The model under review builds one solid part; all positions refer to its coordinate system, in mm. A direction names the side the tool comes from. Round coordinates to 2 decimals unless told otherwise and drop trailing zeros. Order: outer loops, then holes, each group sorted by start corner. A loop starts at its lowest first (then second) coordinate and runs counter-clockwise, first axis right, second up.
Autodesk Inventor part; units mm, degrees
ref_plane "YZ Plane" through (0, 0, 0) normal (1, 0, 0) x (0, 1, 0)
ref_plane "XZ Plane" through (0, 0, 0) normal (0, 1, 0) x (-1, 0, 0)
ref_plane "XY Plane" through (0, 0, 0) normal (0, 0, 1) x (1, 0, 0)
sketch "Эскиз1" plane through (0, 0, 0) normal (0, 1, 0) x (-1, 0, 0)
  circle A0 centre (0, 8.5) radius 1.3
  circle A1 centre (0, -8.5) radius 1.3
  line L0 (0, 5.7) -> (3, 5.7)
  line L1 (3, 5.7) -> (3, 11.7)
  line L2 (3, 11.7) -> (-10, 11.7)
  line L3 (-10, 11.7) -> (-10, 0)
  line L4 (5.8356, 0) -> (-16.6075, 0) construction
  line L5 (0, 5.7) -> (0, 0)
  circle A2 centre (0, -8.5) radius 1.3
  line L6 (0, -5.7) -> (3, -5.7)
  line L7 (3, -5.7) -> (3, -11.7)
  line L8 (3, -11.7) -> (-10, -11.7)
  line L9 (-10, -11.7) -> (-10, 0)
  line L10 (0, -5.7) -> (0, 0)
  dimension "d1" = 2.6
  dimension "d2" = 2.6
  dimension "d5" = 3
  dimension "d6" = 6
  dimension "d7" = 13
extrude "Выдавливание1" add sketch "Эскиз1" along normal blind 11
fillet "Сопряжение1" radius 2 4 edges at (10, 5.5, 11.7) (-3, 5.5, 11.7) (10, 5.5, -11.7) (-3, 5.5, -11.7)
properties part number "стойки для драйверов"
(1) Consider section C-C (z = 3.25). Write out the cut boundary in (x, y).
Data:
outline: (0, 0) - (10, 0) - (10, 11) - (0, 11) - close
(2) For faces 1 (the flat face through (3, 5, -11.7)), 2 (the flat face through (0, 5, 0)), list the 3-axis set-ups (+Z, -Z, +X, -X, +Y, -Y) from which the entire face can be reached by the end or side of a thin tool; tool diameter is ignored.
Data:
face 1: -Z, +X, -X, +Y, -Y
face 2: -X, +Y, -Y
(3) Draft analysis for pull direction X (two halves, no side actions). For faces 3 (the flat face through (-3, 5, -8)), 4 (the cylindrical face through (0.17, 5.42, -9.79)), 5 (the flat face through (-1, 5, 5.7)), state which applies: pulls with the +X half, pulls with the -X half, needs draft (parallel to the pull), parting line crosses it, or undercut.
Data:
face 3: pulls with the -X half
face 4: undercut
face 5: needs draft
(4) Insertion check: pin 1 (3.5 mm diameter, centred on x = 0, z = -8.5, fed in from -Y). The pin has a flat end and moves straight along its axis. Give the tip position at first contact, or say it passes through.
Data:
pin 1: stops at y = 0
(5) To check wall thickness, follow probe 1 along Z at (x, y) = (-0.5, 5); probe 2 along X at (y, z) = (10.25, 1.5); probe 3 along X at (y, z) = (4.25, 7.75). State the ranges of each line that lie inside material, in increasing order.
Data:
probe 1: z = -11.7 to -9.7, -7.3 to -5.7, 5.7 to 7.3, 9.7 to 11.7
probe 2: x = 0 to 10
probe 3: x = -3 to -1.06, 1.06 to 10
(6) Consider section A-A (z = 8.5). Write out the cut boundary in (x, y).
Data:
outline: (-3, 0) - (-1.3, 0) - (-1.3, 11) - (-3, 11) - close; (1.3, 0) - (10, 0) - (10, 11) - (1.3, 11) - close
(7) Consider section B-B (y = 2.5). Write out the cut boundary in (x, z).
Data:
outline: (-3, -9.7) arc R2 ccw to (-1, -11.7) - (8, -11.7) arc R2 ccw to (10, -9.7) - (10, 9.7) arc R2 ccw to (8, 11.7) - (-1, 11.7) arc R2 ccw to (-3, 9.7) - (-3, 5.7) - (0, 5.7) - (0, -5.7) - (-3, -5.7) - close; hole circle Ø2.6 at (0, -8.5); hole circle Ø2.6 at (0, 8.5)
